```python
from build123d import *

# Parameters (mm, degrees)
SKETCH1_R             = 14
SKETCH1_R_2           = 11.1125
BOSS_EXTRUDE1_DEPTH   = 3.175
F_6_CLEARANCE_HOLE1_D = 3.6576
M4_CLEARANCE_HOLE1_D  = 4.3


with BuildPart() as part:
    # Sketch1 → Boss-Extrude1 (new, symmetric)
    with BuildSketch(Plane(origin=(0, 0, 0), x_dir=(0, 0, -1), z_dir=(1, 0, 0))):
        with BuildLine():
            Line((-133.81, -16.645), (-94.632187648, -66.087166556))
            ThreePointArc((-94.632187648, -66.087166556), (-72.998034274, -77.560353063), (-49.900079745, -69.426774672))
            Line((-49.900079745, -69.426774672), (11.366191703, -12.160004571))
            ThreePointArc((11.366191703, -12.160004571), (15.483205435, 6.109531443), (0, 16.645))
            Line((0, 16.645), (-133.81, 16.645))
            Line((-133.81, 16.645), (-133.81, -16.645))
        make_face()
        with Locations((-70.72728593, -47.145)):
            Circle(SKETCH1_R, mode=Mode.SUBTRACT)
        Circle(SKETCH1_R_2, mode=Mode.SUBTRACT)
    extrude(amount=BOSS_EXTRUDE1_DEPTH, both=True)

    # #6 Clearance Hole1 (through all)
    with Locations(Plane(origin=(3.175, 0, 0), x_dir=(0, 0, -1), z_dir=(1, 0, 0))):
        with Locations((-80, -13.475), (-80, 13.475), (-130, 13.475), (-130, -13.475)):
            Hole(F_6_CLEARANCE_HOLE1_D / 2)

    # M4 Clearance Hole1 (through all)
    with Locations(Plane(origin=(3.175, 0, 0), x_dir=(0, 0, -1), z_dir=(1, 0, 0))):
        with Locations((-72.109641, -25.689485686), (-88.617128841, -59.069911765), (-51.455087948, -56.675602549)):
            Hole(M4_CLEARANCE_HOLE1_D / 2)


solid = part.part
```
Read the model definition and answer for the solid it produces. Units are mm, in the model's axes. Round coordinates to 2 decimals unless told otherwise and drop trailing zeros. Write each loop counter-clockwise with the first axis right and the second up, starting at its lowest first coordinate (ties: lowest second). Pieces come first, ordered by that corner, then holes. Notation, with made-up numbers: (59.25, 57) - (97.25, 57) arc R12 ccw to (97.25, 72) - close; hole circle Ø10 at (-26, -20.5). An arc over 180 degrees is marked (long way). One line per item, written item: value.
Q1. Straight lines are drawn through the part: line 1 (Y direction, x = 0.25, z = 80) (3 decimals); line 2 (Z direction, x = 2.5, y = -58); line 3 (Z direction, x = 0.75, y = -60). For each, find the intervals that lie inside material, in ascending order. Write a range as from..to.
The answers:
line 1: y = -76.201..-57.634, -36.656..-15.304, -11.646..11.646, 15.304..16.645
line 2: z = 37.68..49.76, 53.15..61.89, 79.57..86.75, 90.48..101.04
line 3: z = 39.81..65.18, 76.27..86.68, 90.56..99.46
Q2. This flat-tipped pin is pushed along its axis until it touches: P1, Ø1.5, axis at x = 1, z = 80, coming from the -Y side. Where does it stop, or does it pass through?
The answers:
P1: stops at y = -76.43
Q3. For a pull along Y with two mould halves and no side action, classify faces 1 (the flat face through (-3.175, -19, 60)), 2 (the cylindrical face through (-0.044, -12.926, 131.744)), 3 (the flat face through (0, 16.645, 66)), 4 (the flat face through (0.044, -41.02, 114.495)) as pulls with the +Y half, pulls with the -Y half, needs draft (parallel to the pull), parting line crosses it, or undercut.
The answers:
face 1: needs draft
face 2: undercut
face 3: pulls with the +Y half
face 4: pulls with the -Y half
Q4. Find section B-B (z = 130). Determine the outline of the cut face in (x, y) (3 decimals).
The answers:
outline: (-3.175, -21.453) - (3.175, -21.453) - (3.175, -15.304) - (-3.175, -15.304) - close; (-3.175, -11.646) - (3.175, -11.646) - (3.175, 11.646) - (-3.175, 11.646) - close; (-3.175, 15.304) - (3.175, 15.304) - (3.175, 16.645) - (-3.175, 16.645) - close
Q5. Find section D-D (z = 104.5). Determine the outline of the cut face in (x, y) (3 decimals).
The answers:
outline: (-3.175, -53.634) - (3.175, -53.634) - (3.175, 16.645) - (-3.175, 16.645) - close
Q6. Find section C-C (x = -0.75). Count the separate pieces of the cut face and the enclosed holes in it, and give its area (3 significant figures).
The answers:
separate pieces: 1
enclosed holes: 9
area: 8,860 mm2
Q7. Find section A-A (y = 0). Determine the outline of the cut face in (x, z) (1 decimal), and give its area (3 significant figures).
The answers:
outline: (-3.2, -16.6) - (3.2, -16.6) - (3.2, -11.1) - (-3.2, -11.1) - close; (-3.2, 11.1) - (3.2, 11.1) - (3.2, 133.8) - (-3.2, 133.8) - close
area: 814 mm2
